```python
from build123d import *

# Parameters (mm, degrees)
F1_DEPTH = 75
F3_DEPTH = 5
F5_DEPTH = 5
F6_R     = 1.5
F7_DEPTH = 5


with BuildPart() as f1:
    # F0 (on Right) → F1 (new body)
    with BuildSketch(Plane.YZ):
        Polygon((70, 0), (0, 0), (0, -5), (75, -5), (75, 70), (70, 70), align=None)
    extrude(amount=F1_DEPTH)

    # F2 (on face) → F3 (join)
    with BuildSketch(Plane.YZ.offset(75)):
        Polygon((70, 0), (70, 70), (0, 0), align=None)
    extrude(amount=-F3_DEPTH)

    # F4 (on face) → F5 (join)
    with BuildSketch(Plane(origin=(0, 0, 0), x_dir=(0, -1, 0), z_dir=(-1, 0, 0))):
        Polygon((-70, 70), (-70, 0), (0, 0), align=None)
    extrude(amount=-F5_DEPTH)

    # F6 (on face) → F7 (cut, through all)
    with BuildSketch(Plane(origin=(0, 75, 0), x_dir=(-1, 0, 0), z_dir=(0, 1, 0))):
        with Locations((-65, 26)):
            Circle(F6_R)
        with Locations((-49.75, 26)):
            Circle(F6_R)
        with Locations((-49.75, 5)):
            Circle(F6_R)
        with Locations((-65, 5)):
            Circle(F6_R)
        with Locations((-10, 5)):
            Circle(F6_R)
        with Locations((-25.25, 5)):
            Circle(F6_R)
        with Locations((-25.25, 26)):
            Circle(F6_R)
        with Locations((-10, 26)):
            Circle(F6_R)
    extrude(amount=-F7_DEPTH, mode=Mode.SUBTRACT)


solid = f1.part
```
The model under review builds one solid part; all positions refer to its coordinate system, in mm. A direction names the side the tool comes from. Round coordinates to 2 decimals unless told otherwise and drop trailing zeros. Order: outer loops, then holes, each group sorted by start corner. A loop starts at its lowest first (then second) coordinate and runs counter-clockwise, first axis right, second up. Notation, with made-up numbers: M 20.5,-3 L 59.5,-3 A28 cw 59.5,19 Z; hole C 88.25,86 d9. An arc over 180 degrees is marked long. Use a Markdown table: item, result.
1) Tool access review of faces 5 (the face through (5, 51, 20)), 6 (the face through (50.86, 72.54, 27.01)): name each direction out of +Z, -Z, +X, -X, +Y, -Y from which nothing blocks a thin tool from reaching the whole face with its end or side.
Report:
| item | result |
|---|---|
| face 5 | +Z, -Y |
| face 6 | +Y, -Y |
2) Consider section B-B (x = 65). Write out the cut boundary in (y, z), then the cut area to 3 significant figures.
Report:
| item | result |
|---|---|
| outline | M 0,-5 L 75,-5 L 75,3.5 L 70,3.5 L 70,0 L 0,0 Z; M 70,6.5 L 75,6.5 L 75,24.5 L 70,24.5 Z; M 70,27.5 L 75,27.5 L 75,70 L 70,70 Z |
| area | 695 mm^2 |
3) Insertion check: pin 1 (2 mm diameter, centred on x = 24.5, z = 5.5, fed in from -Y); pin 2 (2.5 mm diameter, centred on x = 25.25, z = 5, fed in from +Y); pin 3 (8 mm diameter, centred on x = 49.5, y = 50, fed in from +Z). Each pin has a flat end and moves straight along its axis. Give the tip position at first contact, or say it passes through.
Report:
| item | result |
|---|---|
| pin 1 | y = 70 |
| pin 2 | through |
| pin 3 | z = 0 |
4) Consider section A-A (z = 26). Write out the cut boundary in (x, y), then the cut area to 3 significant figures.
Report:
| item | result |
|---|---|
| outline | M 0,26 L 5,26 L 5,70 L 8.5,70 L 8.5,75 L 0,75 Z; M 11.5,70 L 23.75,70 L 23.75,75 L 11.5,75 Z; M 26.75,70 L 48.25,70 L 48.25,75 L 26.75,75 Z; M 51.25,70 L 63.5,70 L 63.5,75 L 51.25,75 Z; M 66.5,70 L 70,70 L 70,26 L 75,26 L 75,75 L 66.5,75 Z |
| area | 755 mm^2 |
5) Wall thickness on line 1 along Z through (x, y) = (10, 71.9); line 2 along X through (y, z) = (45, 14.5); line 3 along Z through (x, y) = (25, 65): over which ranges is each line inside the solid? List them lowest first. Write a range as [from, to].
Report:
| item | result |
|---|---|
| line 1 | [-5, 3.5], [6.5, 24.5], [27.5, 70] |
| line 2 | [0, 5], [70, 75] |
| line 3 | [-5, 0] |
6) Consider section D-D (x = 17.5). Write out the cut boundary in (y, z), then the cut area to 3 significant figures.
Report:
| item | result |
|---|---|
| outline | M 0,-5 L 75,-5 L 75,70 L 70,70 L 70,0 L 0,0 Z |
| area | 725 mm^2 |
7) Consider section C-C (y = 25). Write out the cut boundary in (x, z).
Report:
| item | result |
|---|---|
| outline | M 0,-5 L 75,-5 L 75,25 L 70,25 L 70,0 L 5,0 L 5,25 L 0,25 Z |
8) Draft analysis for pull direction X (two halves, no side actions). For faces 1 (the face through (63.57, 72.54, 5.45)), 2 (the face through (0, 46, 25)), 3 (the face through (75, 45, 25)), 4 (the face through (37, 37, -5)), state which applies: released by +X, released by -X, zero draft, split by the parting line, or undercut.
Report:
| item | result |
|---|---|
| face 1 | undercut |
| face 2 | released by -X |
| face 3 | released by +X |
| face 4 | zero draft |
